Check sheet for the modelled part. Datum: model origin and axes. Units: mm. Give positions to 0.01 mm unless a question says otherwise; leave off trailing zeros. Order: outer loops, then holes, each group sorted by start corner. A loop starts at its lowest first (then second) coordinate and runs counter-clockwise, first axis right, second up.
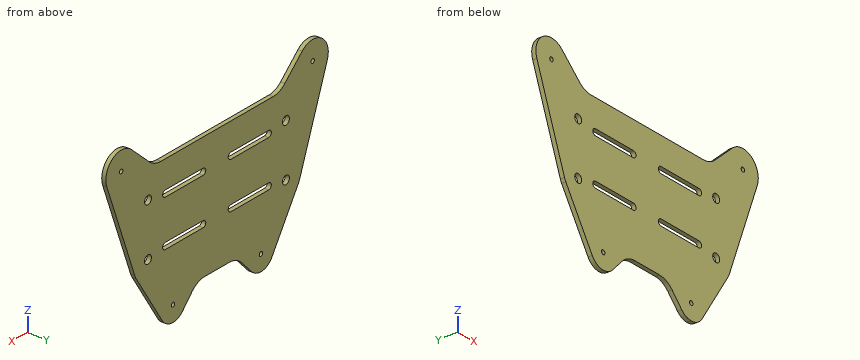
from build123d import *

# Parameters (mm, degrees)
SKETCH1_W           = 130
SKETCH1_H           = 90
BOSS_EXTRUDE2_DEPTH = 2
SKETCH2_R           = 2
CUT_EXTRUDE1_DEPTH  = 10
CUT_EXTRUDE3_DEPTH  = 10
SKETCH5_R           = 1
CUT_EXTRUDE4_DEPTH  = 10
CUT_EXTRUDE5_DEPTH  = 3
FILLET1_R           = 10


with BuildPart() as part:
    # Sketch1 → Boss-Extrude2 (new body)
    with BuildSketch(Plane(origin=(0, 0, 0), x_dir=(1, 0, 0), z_dir=(0, 1, 0))):
        with Locations((56.787418592, 40.403463793)):
            Rectangle(SKETCH1_W, SKETCH1_H)
    extrude(amount=BOSS_EXTRUDE2_DEPTH)

    # Sketch2 → Cut-Extrude1 (cut)
    with BuildSketch(Plane(origin=(0, 2, 0), x_dir=(1, 0, 0), z_dir=(0, 1, 0))):
        with Locations((16.787418592, 52.903463793)):
            Circle(SKETCH2_R)
        with Locations((16.787418592, 27.903463793)):
            Circle(SKETCH2_R)
        with Locations((96.787418592, 52.903463793)):
            Circle(SKETCH2_R)
        with Locations((96.787418592, 27.903463793)):
            Circle(SKETCH2_R)
    extrude(amount=-CUT_EXTRUDE1_DEPTH, mode=Mode.SUBTRACT)

    # Sketch4 → Cut-Extrude3 (cut)
    with BuildSketch(Plane(origin=(0, 2, 0), x_dir=(1, 0, 0), z_dir=(0, 1, 0))):
        with BuildLine():
            Line((26.787418592, 52.903463793), (48.787418592, 52.903463793))
            ThreePointArc((48.787418592, 52.903463793), (50.287418592, 51.403463793), (48.787418592, 49.903463793))
            Line((48.787418592, 49.903463793), (26.787418592, 49.903463793))
            ThreePointArc((26.787418592, 49.903463793), (25.287418592, 51.403463793), (26.787418592, 52.903463793))
        make_face()
        with BuildLine():
            Line((26.787418592, 30.903463793), (48.787418592, 30.903463793))
            ThreePointArc((48.787418592, 30.903463793), (50.287418592, 29.403463793), (48.787418592, 27.903463793))
            Line((48.787418592, 27.903463793), (26.787418592, 27.903463793))
            ThreePointArc((26.787418592, 27.903463793), (25.287418592, 29.403463793), (26.787418592, 30.903463793))
        make_face()
        with BuildLine():
            Line((64.787418592, 52.903463793), (86.787418592, 52.903463793))
            ThreePointArc((86.787418592, 52.903463793), (88.287418592, 51.403463793), (86.787418592, 49.903463793))
            Line((86.787418592, 49.903463793), (64.787418592, 49.903463793))
            ThreePointArc((64.787418592, 49.903463793), (63.287418592, 51.403463793), (64.787418592, 52.903463793))
        make_face()
        with BuildLine():
            Line((64.787418592, 30.903463793), (86.787418592, 30.903463793))
            ThreePointArc((86.787418592, 30.903463793), (88.287418592, 29.403463793), (86.787418592, 27.903463793))
            Line((86.787418592, 27.903463793), (64.787418592, 27.903463793))
            ThreePointArc((64.787418592, 27.903463793), (63.287418592, 29.403463793), (64.787418592, 30.903463793))
        make_face()
    extrude(amount=-CUT_EXTRUDE3_DEPTH, mode=Mode.SUBTRACT)

    # Sketch5 → Cut-Extrude4 (cut)
    with BuildSketch(Plane(origin=(0, 2, 0), x_dir=(1, 0, 0), z_dir=(0, 1, 0))):
        with Locations((1.287418592, 9.403463793)):
            Circle(SKETCH5_R)
        with Locations((112.287418592, 9.403463793)):
            Circle(SKETCH5_R)
        with Locations((31.287418592, 77.903463793)):
            Circle(SKETCH5_R)
        with Locations((82.287418592, 77.903463793)):
            Circle(SKETCH5_R)
    extrude(amount=-CUT_EXTRUDE4_DEPTH, mode=Mode.SUBTRACT)

    # Sketch6 → Cut-Extrude5 (cut, through all)
    with BuildSketch(Plane(origin=(0, 2, 0), x_dir=(1, 0, 0), z_dir=(0, 1, 0))):
        with BuildLine():
            Line((31.287418742, 85.403463793), (-8.212581408, 85.403463793))
            Line((-8.212581408, 85.403463793), (-8.212581408, -4.596536207))
            Line((-8.212581408, -4.596536207), (121.787418592, -4.596536207))
            Line((121.787418592, -4.596536207), (121.787418592, 85.403463793))
            Line((121.787418592, 85.403463793), (82.287418592, 85.403463793))
            ThreePointArc((82.287418592, 85.403463793), (85.908182742, 84.471573641), (88.629172371, 81.907481652))
            Line((88.629172371, 81.907481652), (104.107184656, 57.392670192))
            Line((104.107184656, 57.392670192), (120.652052771, 12.485171021))
            ThreePointArc((120.652052771, 12.485171021), (117.254615926, 2.001371181), (106.265325845, 2.830913046))
            Line((106.265325845, 2.830913046), (93.195977552, 14.805689748))
            Line((93.195977552, 14.805689748), (20.378859632, 14.805689748))
            Line((20.378859632, 14.805689748), (7.425097101, 2.787815466))
            ThreePointArc((7.425097103, 2.787815464), (-3.723088928, 1.897951505), (-7.176040156, 12.53519915))
            Line((-7.176040154, 12.53519915), (8.848458195, 55.841119114))
            ThreePointArc((8.848458195, 55.841119114), (9.189915505, 56.63640604), (9.610794254, 57.392670192))
            Line((9.610794254, 57.392670192), (24.928951385, 81.880886929))
            ThreePointArc((24.928951386, 81.880886928), (27.652908616, 84.463977282), (31.287418742, 85.403463793))
        make_face()
        with BuildLine():
            Line((82.287418592, 85.403463793), (31.287418742, 85.403463793))
            ThreePointArc((31.287418742, 85.403463793), (34.283566796, 84.779007113), (36.780790962, 83.00962282))
            Line((36.780790963, 83.009622821), (45.361476392, 73.77824166))
            Line((45.361476392, 73.77824166), (68.213360792, 73.77824166))
            Line((68.213360792, 73.77824166), (76.794046223, 83.009622821))
            ThreePointArc((76.794046223, 83.009622821), (79.291270457, 84.779007143), (82.287418592, 85.403463793))
        make_face()
    extrude(amount=-CUT_EXTRUDE5_DEPTH, mode=Mode.SUBTRACT)

    # Fillet1
    fillet1_edges = [part.edges().sort_by_distance(p)[0] for p in [
        (68.213360792, 1, -73.77824166),
        (45.361476392, 1, -73.77824166),
        (20.378859632, 1, -14.805689748),
        (93.195977552, 1, -14.805689748),
        (104.107184656, 1, -57.392670192),
    ]]
    fillet(fillet1_edges, radius=FILLET1_R)


solid = part.part
1) Material ranges on L1, parallel to X at y = 0.75, z = -51.5; L2, parallel to Z at x = 83.5, y = 1.3; L3, parallel to Z at x = 44.5, y = 0.25, recorded low to high.
Recorded:
L1: x = 7.24 to 15.36, 18.21 to 25.29, 50.28 to 63.29, 88.28 to 95.36, 98.21 to 106.28
L2: z = -85.3 to -52.9, -49.9 to -30.9, -27.9 to -14.81
L3: z = -75.25 to -52.9, -49.9 to -30.9, -27.9 to -14.81
2) Section check D-D, the plane y = 0.5. State how many separate pieces and enclosed holes the cut face has, then the cut area to 3 significant figures.
Recorded:
separate pieces: 1
enclosed holes: 12
area: 6,650 mm2
3) Section check C-C, the plane x = 61. Record the cut outline in (y, z).
Recorded:
outline: (0, -73.78) - (2, -73.78) - (2, -14.81) - (0, -14.81) - close
4) Section check A-A, the plane x = 78.5. Record the cut outline in (y, z), then the cut area to 3 significant figures.
Recorded:
outline: (0, -84.38) - (2, -84.38) - (2, -52.9) - (0, -52.9) - close; (0, -49.9) - (2, -49.9) - (2, -30.9) - (0, -30.9) - close; (0, -27.9) - (2, -27.9) - (2, -14.81) - (0, -14.81) - close
area: 127 mm2
5) Depth check by flat-ended pin: pin 1 Ø0.6 at (x, y) = (80, 1) entering from +Z; pin 2 Ø3 at (x, z) = (96.79, -27.9) entering from -Y; pin 3 Ø1 at (x, y) = (47.5, 0.5) entering from -Z; pin 4 Ø1 at (x, y) = (40, 1.5) entering from -Z. Enter the tip coordinate at first touch or a pass-through.
Recorded:
pin 1: stops at z = -14.81
pin 2: passes through
pin 3: stops at z = -74.16
pin 4: stops at z = -80.08
6) Section check B-B, the plane z = -47. Record the cut outline in (x, y).
Recorded:
outline: (5.58, 0) - (107.94, 0) - (107.94, 2) - (5.58, 2) - close
